from build123d import *

# Parameters (mm, degrees)
F2_R     = 6.75
F3_DEPTH = 9
F4_R     = 3.5
F5_DEPTH = 25.001


with BuildPart() as f1:
    # F0 (on Right) → F1 (revolve)
    with BuildSketch(Plane.YZ):
        Polygon((3.3, 16), (32, 16), (32, 36), (25, 36), (25, 82.5), (0, 82.5), (0, 65), (3.3, 65), align=None)
    revolve(axis=Axis((0, 21.725982, 0), (0, 1, 0)))

    # F2 (on face) → F3 (cut)
    with BuildSketch(Plane.XZ.offset(-3.3)):
        with Locations((0, 42)):
            Circle(F2_R)
        with Locations((36.373067, -21)):
            Circle(F2_R)
        with Locations((-36.373067, -21)):
            Circle(F2_R)
    extrude(amount=-F3_DEPTH, mode=Mode.SUBTRACT)

    # F4 (on face) → F5 (cut, through all)
    with BuildSketch(Plane(origin=(0, 25, 0), x_dir=(-1, 0, 0), z_dir=(0, 1, 0))):
        with Locations((0, 42)):
            Circle(F4_R)
        with Locations((-36.373067, -21)):
            Circle(F4_R)
        with Locations((36.373067, -21)):
            Circle(F4_R)
    extrude(amount=-F5_DEPTH, mode=Mode.SUBTRACT)


solid = f1.part
Geometry check sheet. Reference: the model listing, model coordinates, mm. A direction names the side the tool comes from. Round coordinates to 2 decimals unless told otherwise and drop trailing zeros. Write each loop counter-clockwise with the first axis right and the second up, starting at its lowest first coordinate (ties: lowest second). Pieces come first, ordered by that corner, then holes.
Item 1: Section check D-D (z = -21). Record the boundary of the cut face in (x, y), plus the area to 3 significant figures.
Determined:
outline: (-79.78, 0) - (-61.51, 0) - (-61.51, 3.3) - (-43.12, 3.3) - (-43.12, 12.3) - (-39.87, 12.3) - (-39.87, 25) - (-79.78, 25) - close; (-32.87, 12.3) - (-29.62, 12.3) - (-29.62, 3.3) - (29.62, 3.3) - (29.62, 12.3) - (32.87, 12.3) - (32.87, 25) - (29.24, 25) - (29.24, 32) - (-29.24, 32) - (-29.24, 25) - (-32.87, 25) - close; (39.87, 12.3) - (43.12, 12.3) - (43.12, 3.3) - (61.51, 3.3) - (61.51, 0) - (79.78, 0) - (79.78, 25) - (39.87, 25) - close
area: 3,570 mm2
Item 2: Go/stop test with flat-tipped pins: pin 1 Ø1.5 at (x, y) = (-7, 10) entering from +Z; pin 2 Ø15.5 at (x, z) = (0, 42) entering from -Y; pin 3 Ø3 at (y, z) = (14, -35) entering from -X. Record where each tip stops, or that it passes through.
Determined:
pin 1: stops at z = 82.26
pin 2: stops at y = 3.3
pin 3: stops at x = -75.39
Item 3: Access from +Z, -Z, +X, -X, +Y, -Y to the whole of each face (thin tool, end or side, straight path). Record for faces 4 (the face through (3, 12.3, 39)), 5 (the face through (-15.62, 17.85, -3.47)).
Determined:
face 4: -Y
face 5: +Y, -Y
Item 4: Section check B-B (z = 0). Record the boundary of the cut face in (x, y), plus the area to 3 significant figures.
Determined:
outline: (-82.5, 0) - (-65, 0) - (-65, 3.3) - (-16, 3.3) - (-16, 32) - (-36, 32) - (-36, 25) - (-82.5, 25) - close; (16, 3.3) - (65, 3.3) - (65, 0) - (82.5, 0) - (82.5, 25) - (36, 25) - (36, 32) - (16, 32) - close
area: 3,280 mm2
Item 5: Mould release check, pull along X, two halves, no side actions. Record for faces 1 (the face through (35.694, 28.451, -4.686)), 2 (the face through (29.63, 7.74, -20.7)), 3 (the face through (-17, 25, -36)): +X half, -X half, draft (parallel to the pull), parting line (faces both ways), or undercut.
Determined:
face 1: parting line
face 2: undercut
face 3: draft
Item 6: Section check C-C (y = 8.5). Record the boundary of the cut face in (x, z), plus the area to 3 significant figures.
Determined:
outline: circle Ø165 at (0, 0); hole circle Ø13.5 at (-36.37, -21); hole circle Ø32 at (0, 0); hole circle Ø13.5 at (0, 42); hole circle Ø13.5 at (36.37, -21)
area: 20,100 mm2
Item 7: Material ranges on line 1 along X through (y, z) = (2, 0); line 2 along X through (y, z) = (4, -16.5); line 3 along Y through (x, z) = (22.5, 13.5), recorded low to high.
Determined:
line 1: x = -82.5 to -65, 65 to 82.5
line 2: x = -80.83 to -41.4, -31.34 to 31.34, 41.4 to 80.83
line 3: y = 3.3 to 32
Item 8: Section check A-A (x = 0). Record the boundary of the cut face in (y, z).
Determined:
outline: (0, -82.5) - (25, -82.5) - (25, -36) - (32, -36) - (32, -16) - (3.3, -16) - (3.3, -65) - (0, -65) - close; (0, 65) - (3.3, 65) - (3.3, 48.75) - (12.3, 48.75) - (12.3, 45.5) - (25, 45.5) - (25, 82.5) - (0, 82.5) - close; (3.3, 16) - (32, 16) - (32, 36) - (25, 36) - (25, 38.5) - (12.3, 38.5) - (12.3, 35.25) - (3.3, 35.25) - close
